from build123d import *

# Parameters (mm, degrees)
CROQUIS1_W              = 54.5
CROQUIS1_H              = 35
SALIENTE_EXTRUIR1_DEPTH = 7.85
SALIENTE_EXTRUIR2_DEPTH = 35
CROQUIS3_W              = 54.5
CROQUIS3_H              = 7.85
SALIENTE_EXTRUIR3_DEPTH = 15
CROQUIS4_W              = 1.5
CROQUIS4_H              = 34.809371379
SALIENTE_EXTRUIR4_DEPTH = 4.55
CROQUIS5_W              = 34.809371379
CROQUIS5_H              = 1.5
SALIENTE_EXTRUIR5_DEPTH = 2.85
TALADRO1_AT_2_COUNT     = 2
TALADRO1_AT_2_PITCH     = 40
TALADRO1_AT_3_COUNT     = 2
TALADRO1_AT_3_PITCH     = 20
TALADRO1_AT_4_COUNT     = 2
TALADRO1_AT_4_PITCH     = 20
CHAFL_N1_SIZE           = 1
CROQUIS11_R             = 1.75
SALIENTE_EXTRUIR6_DEPTH = 3
CHAFL_N2_SIZE           = 1


with BuildPart() as part:
    # Croquis1 → Saliente-Extruir1 (new body)
    with BuildSketch(Plane.XZ.offset(-3.05)):
        with Locations((22.9, 8)):
            Rectangle(CROQUIS1_W, CROQUIS1_H)
    extrude(amount=-SALIENTE_EXTRUIR1_DEPTH)

    # Croquis2 → Saliente-Extruir2 (add)
    with BuildSketch(Plane.XY.offset(25.5)):
        Polygon((-4.35, 3.05), (-4.35, -1.5), (0, -1.5), (0, 0), (-2.85, 0), (-2.85, 3.05), align=None)
    extrude(amount=-SALIENTE_EXTRUIR2_DEPTH)

    # Croquis3 → Saliente-Extruir3 (add)
    with BuildSketch(Plane.XY.offset(25.5)):
        with Locations((22.9, 6.975)):
            Rectangle(CROQUIS3_W, CROQUIS3_H)
    extrude(amount=SALIENTE_EXTRUIR3_DEPTH)

    # Croquis4 → Saliente-Extruir4 (add)
    with BuildSketch(Plane.XZ.offset(-3.05)):
        with Locations((49.4, 7.90468569)):
            Rectangle(CROQUIS4_W, CROQUIS4_H)
    extrude(amount=SALIENTE_EXTRUIR4_DEPTH)

    # Croquis5 → Saliente-Extruir5 (add)
    with BuildSketch(Plane.ZY.offset(-48.65)):
        with Locations((7.90468569, -0.75)):
            Rectangle(CROQUIS5_W, CROQUIS5_H)
    extrude(amount=SALIENTE_EXTRUIR5_DEPTH)

    # Croquis7 → Taladro1 (revolve, cut)
    with BuildSketch(Plane(origin=(2.9, 3.05, 2.5), x_dir=(0, 0, -1), z_dir=(1, 0, 0))):
        Polygon((0, 0), (0, 7.85), (3, 7.85), (3, 3.15), (4.5, 3.15), (4.5, 0), align=None)
    taladro1 = revolve(axis=Axis((2.9, 113.05, 2.5), (0, -1, 0)), mode=Mode.SUBTRACT)

    # Taladro1 at 2: Taladro1 ×2
    with Locations(*[(i * TALADRO1_AT_2_PITCH, 0, 0) for i in range(1, TALADRO1_AT_2_COUNT)]):
        add(taladro1, mode=Mode.SUBTRACT)

    # Taladro1 at 3: Taladro1 ×2
    with Locations(*[(i * TALADRO1_AT_3_PITCH, 0, 0) for i in range(1, TALADRO1_AT_3_COUNT)]):
        add(taladro1, mode=Mode.SUBTRACT)

    # Taladro1 at 4: Taladro1 ×2
    with Locations(*[(0, 0, i * TALADRO1_AT_4_PITCH) for i in range(1, TALADRO1_AT_4_COUNT)]):
        add(taladro1, mode=Mode.SUBTRACT)

    # Croquis9 → Taladro2 (revolve, cut)
    with BuildSketch(Plane(origin=(42.9, 3.05, 22.5), x_dir=(0, 0, -1), z_dir=(1, 0, 0))):
        Polygon((0, 0), (0, 7.85), (3, 7.85), (3, 4.65), (4.5, 3.15), (4.5, 0), align=None)
    revolve(axis=Axis((42.9, -3.080023899, 22.5), (0, 1, 0)), mode=Mode.SUBTRACT)

    # Chaflán1
    chafl_n1_edges = [part.edges().sort_by_distance(p)[0] for p in [
        (2.9, 6.2, 25.5),
        (22.9, 6.2, 5.5),
        (42.9, 6.2, 5.5),
        (2.9, 6.2, 5.5),
    ]]
    chamfer(chafl_n1_edges, length=CHAFL_N1_SIZE)

    # Croquis11 → Saliente-Extruir6 (add)
    with BuildSketch(Plane(origin=(0, 0, -9.5), x_dir=(-1, 0, 0), z_dir=(0, 0, -1))):
        with BuildLine():
            Line((-50.15, 10.9), (4.35, 10.9))
            Line((4.35, 10.9), (4.35, -29.1))
            Line((4.35, -29.1), (-3.985719681, -29.1))
            ThreePointArc((-3.985719681, -29.1), (-22.9, -15.6), (-41.814280319, -29.1))
            Line((-41.814280319, -29.1), (-50.15, -29.1))
            Line((-50.15, -29.1), (-50.15, 10.9))
        make_face()
        with Locations((-38.4, -14.95)):
            Circle(CROQUIS11_R, mode=Mode.SUBTRACT)
        with Locations((-7.4, -14.95)):
            Circle(CROQUIS11_R, mode=Mode.SUBTRACT)
    extrude(amount=-SALIENTE_EXTRUIR6_DEPTH)

    # Chaflán2
    chafl_n2_edges = [part.edges().sort_by_distance(p)[0] for p in [
        (40.15, -14.95, -9.5),
        (9.15, -14.95, -9.5),
    ]]
    chamfer(chafl_n2_edges, length=CHAFL_N2_SIZE)


solid = part.part
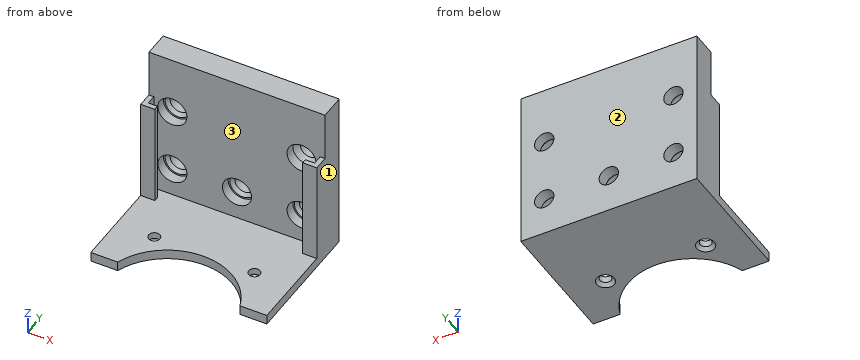
Build history of the part. All positions in model axes, mm. Face numbers are marked on the shaded views. Coordinates: 2 decimals unless noted, no trailing zeros. Write each loop counter-clockwise with the first axis right and the second up, starting at its lowest first coordinate (ties: lowest second). Pieces come first, ordered by that corner, then holes.
(1) Mould opens along X. For the marked faces 1, 2 and 3 say: pulls with the +X half, pulls with the -X half, needs draft (parallel to the pull), parting line crosses it, or undercut.
(2) Pin check, flat tips, straight feed: pin 1 Ø14.5 at (x, z) = (42.9, 2.5) entering from -Y; pin 2 Ø2 at (x, y) = (7, -7) entering from +Z; pin 3 Ø8 at (x, z) = (6, 5.5) entering from -Y. Stop position of each tip, or through.
(3) Cut at A-A on x = 2.9. List the corners of the cut face in (y, z).
(4) Cut at C-C on y = -22. List the corners of the cut face in (x, z).
(5) Cut at D-D on z = 2.5. State how many separate pieces and enclosed holes the cut face has, and give its area (3 significant figures).
(6) Cut at B-B on x = 22.9. List the corners of the cut face in (y, z), and give its area (3 significant figures).
(7) Drill centre lines: line 1 (X direction, y = 8.4, z = 2.5); line 2 (X direction, y = 5.3, z = 2.5); line 3 (X direction, y = 10.05, z = 22.5). Where is each one in solid material? Low to high.
Working result:
1. face 1: pulls with the +X half
1. face 2: needs draft
1. face 3: undercut
2. pin 1: stops at y = -1.5
2. pin 2: stops at z = -6.5
2. pin 3: stops at y = 3.05
3. outline: (-29.1, -9.5) - (10.9, -9.5) - (10.9, -0.5) - (7.2, -0.5) - (6.2, -1.5) - (6.2, -2) - (3.05, -2) - (3.05, -6.5) - (-29.1, -6.5) - close; (3.05, 7) - (6.2, 7) - (6.2, 6.5) - (7.2, 5.5) - (10.9, 5.5) - (10.9, 19.5) - (7.2, 19.5) - (6.2, 18.5) - (6.2, 18) - (3.05, 18) - close; (3.05, 27) - (6.2, 27) - (6.2, 26.5) - (7.2, 25.5) - (10.9, 25.5) - (10.9, 40.5) - (3.05, 40.5) - close
4. outline: (-4.35, -9.5) - (8.24, -9.5) - (8.24, -6.5) - (-4.35, -6.5) - close; (37.56, -9.5) - (50.15, -9.5) - (50.15, -6.5) - (37.56, -6.5) - close
5. separate pieces: 4
5. enclosed holes: 0
5. area: 277 mm2
6. outline: (-15.6, -9.5) - (10.9, -9.5) - (10.9, -0.5) - (7.2, -0.5) - (6.2, -1.5) - (6.2, -2) - (3.05, -2) - (3.05, -6.5) - (-15.6, -6.5) - close; (3.05, 7) - (6.2, 7) - (6.2, 6.5) - (7.2, 5.5) - (10.9, 5.5) - (10.9, 40.5) - (3.05, 40.5) - close
6. area: 391 mm2
7. line 1: x = -4.35 to -0.1, 5.9 to 19.9, 25.9 to 39.9, 45.9 to 50.15
7. line 2: x = -4.35 to -1.6, 7.4 to 18.4, 27.4 to 38.4, 47.4 to 50.15
7. line 3: x = -4.35 to -0.1, 5.9 to 39.9, 45.9 to 50.15
